Check sheet for the modelled part. Datum: model origin and axes. Units: mm. Face numbers are marked on the shaded views. A direction names the side the tool comes from. Give positions to 0.01 mm unless a question says otherwise; leave off trailing zeros. Order: outer loops, then holes, each group sorted by start corner. A loop starts at its lowest first (then second) coordinate and runs counter-clockwise, first axis right, second up. Notation, with made-up numbers: (20.5, -13.75) -> (48.5, -13.75) arc R30 cw to (48.5, 23.25) -> close; hole circle Ø9 at (55, -9). An arc over 180 degrees is marked (long way). One line per question, with ' | ' between items.
```python
from build123d import *

# Parameters (mm, degrees)
F1_DEPTH = 110
F2_W     = 110
F2_H     = 380
F3_DEPTH = 270
F5_DEPTH = 110
F6_W     = 380
F6_H     = 40
F7_DEPTH = 380
F9_DEPTH = 230.001


with BuildPart() as f1:
    # F0 (on Top) → F1 (new body)
    with BuildSketch(Plane.XY):
        with BuildLine():
            Line((380, 0), (0, 0))
            Line((0, 0), (0, -380))
            Line((0, -380), (110, -380))
            Line((110, -380), (380, -380))
            ThreePointArc((380, -380), (190, -190), (380, 0))
        make_face()
        with BuildLine():
            Line((380, -380), (380, 0))
            ThreePointArc((380, 0), (190, -190), (380, -380))
        make_face()
        with BuildLine():
            ThreePointArc((570, -190), (514.3502884254, -55.6497115746), (380, 0))
            Line((380, 0), (380, -380))
            ThreePointArc((380, -380), (514.3502884254, -324.3502884254), (570, -190))
        make_face()
    extrude(amount=F1_DEPTH)

    # F2 (on face) → F3 (join)
    with BuildSketch(Plane.XY.offset(110)):
        with Locations((55, -190)):
            Rectangle(F2_W, F2_H)
    extrude(amount=F3_DEPTH)

    # F4 (on face) → F5 (join)
    with BuildSketch(Plane(origin=(0, 0, 0), x_dir=(0, -1, 0), z_dir=(-1, 0, 0))):
        with BuildLine():
            Line((0, 380), (380, 380))
            ThreePointArc((380, 380), (190, 570), (0, 380))
        make_face()
    extrude(amount=-F5_DEPTH)

    # F6 (on face) → F7 (join)
    with BuildSketch(Plane.XY.offset(110)):
        with Locations((300, -210)):
            Rectangle(F6_W, F6_H)
        with Locations((300, -170)):
            Rectangle(F6_W, F6_H)
    extrude(amount=F7_DEPTH)

    # F8 (on face) → F9 (cut, through all)
    with BuildSketch(Plane.XZ.offset(230)):
        Polygon((490, 490), (110, 490), (490, 110), align=None)
    extrude(amount=-F9_DEPTH, mode=Mode.SUBTRACT)


solid = f1.part
```
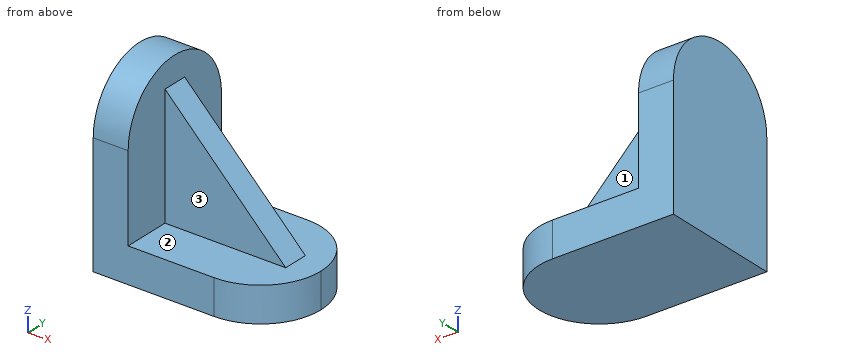
Q1. Depth check by flat-ended pin: pin 1 Ø5 at (x, y) = (242, -246.5) entering from +Z; pin 2 Ø5 at (y, z) = (-328.5, 239) entering from +X; pin 3 Ø1.5 at (x, y) = (446.5, -157) entering from +Z. Enter the tip coordinate at first touch or a pass-through.
Result sheet:
pin 1: stops at z = 110 | pin 2: stops at x = 110 | pin 3: stops at z = 154.25
Q2. Section check D-D (y = -64.5). Enter the section's corners in (x, z).
Result sheet:
outline: (0, 0) -> (522.65, 0) -> (522.65, 110) -> (110, 110) -> (110, 522.65) -> (0, 522.65) -> close
Q3. Section check A-A (x = 262). Enter the section's corners in (y, z), and give its area (3 significant figures).
Result sheet:
outline: (-380, 0) -> (0, 0) -> (0, 110) -> (-150, 110) -> (-150, 338) -> (-230, 338) -> (-230, 110) -> (-380, 110) -> close | area: 60,000 mm2
Q4. Section check B-B (z = 273). Enter the section's corners in (x, y), and give its area (3 significant figures).
Result sheet:
outline: (0, -380) -> (110, -380) -> (110, -230) -> (327, -230) -> (327, -150) -> (110, -150) -> (110, 0) -> (0, 0) -> close | area: 59,200 mm2
Q5. Section check C-C (y = -161). Enter the section's corners in (x, z), and give its area (3 significant figures).
Result sheet:
outline: (0, 0) -> (567.77, 0) -> (567.77, 110) -> (490, 110) -> (110, 490) -> (110, 567.77) -> (0, 567.77) -> close | area: 185,000 mm2
Q6. Access from +Z, -Z, +X, -X, +Y, -Y to the whole of each face (thin tool, end or side, straight path). Record for the marked faces 1, 2 and 3.
Result sheet:
face 1: +Z, +X, +Y | face 2: +Z, +X | face 3: +Z, +X, -Y
Q7. Thickness scan on line 1 (Z direction, x = 370, y = -109); line 2 (Y direction, x = 126, z = 218.5). Record the ranges inside material, lowest first.
Result sheet:
line 1: z = 0 to 110 | line 2: y = -230 to -150
